Can you work these out from the model? Positions are in its coordinate system, mm. A direction names the side the tool comes from. Coordinates: 2 decimals unless noted, no trailing zeros. Order: outer loops, then holes, each group sorted by start corner. A loop starts at its lowest first (then second) coordinate and runs counter-clockwise, first axis right, second up. Notation, with made-up numbers: (78.5, 87.25) -> (121.5, 87.25) arc R20 ccw to (121.5, 98.25) -> close; hole circle Ø10 at (16.25, 42). An arc over 180 degrees is marked (long way). Answer as a JSON object with one key per item and string values. Group by question number.
(1) I want a section at C-C, the plane y = 22.5. List the corners of the cut face in (x, z) for me.
(2) I want a section at D-D, the plane y = 3. List the corners of the cut face in (x, z) for me (3 decimals), plus the area to 3 significant figures.
(3) For pin 1 (1.1 mm diameter, centred on x = 5, z = 4.5, fed in from -Y); pin 2 (0.5 mm diameter, centred on x = 5, z = 4.5, fed in from +Y); pin 3 (3 mm diameter, centred on x = 6, y = 3, fed in from +Z); pin 4 (3 mm diameter, centred on x = 4.5, y = 9.5, fed in from +Z), each with a flat end and sliding along its axis, tell me the tip position at first contact or that it passes through.
(4) I need wall thicknesses on line 1 (Y direction, x = 5, z = 1.65); line 2 (Y direction, x = 5, z = 3.35); line 3 (Y direction, x = 3, z = 1). Which ranges of each line are inside material? Lowest first, please.
(5) If we mould it in two halves opening along X, with no side actions, what happens to faces 6 (the cylindrical face through (9.699, 0.285, 2.028)), 7 (the cylindrical face through (4.792, 30.086, 1.521)), 8 (the flat face through (5, 6, 0))? For each: pulls with the +X half, pulls with the -X half, needs draft (parallel to the pull), parting line crosses it, or undercut.
(6) Which directions (+Z, -Z, +X, -X, +Y, -Y) give clear straight access to the entire face, cutting with the end or side of a thin tool? Please do faces 1 (the flat face through (5, 7, 4)), 2 (the cylindrical face through (5.86, 4.85, 1.52)), 3 (the cylindrical face through (7.586, 2.428, 3.507)), 4 (the cylindrical face through (5.07, 18.535, 0.301)), 5 (the cylindrical face through (9.699, 31.715, 2.028)).
(7) I want a section at B-B, the plane y = 28.5. List the corners of the cut face in (x, z) for me.
(8) I want a section at A-A, the plane x = 5. State how many separate pieces and enclosed holes the cut face has, plus the area to 3 significant figures.
from build123d import *

# Parameters (mm, degrees)
CROQUIS1_W              = 10
CROQUIS1_H              = 32
SALIENTE_EXTRUIR1_DEPTH = 8
CROQUIS2_R              = 1.6
CORTAR_EXTRUIR1_DEPTH   = 8
CROQUIS3_R              = 2.25
CORTAR_EXTRUIR2_DEPTH   = 10
REDONDEO1_R             = 1
CORTAR_EXTRUIR3_START   = -10
CROQUIS4_W              = 4
CROQUIS4_H              = 10
CORTAR_EXTRUIR3_DEPTH   = 10
REDONDEO2_R             = 3
REDONDEO3_R             = 1
CROQUIS5_R              = 2.8
CORTAR_EXTRUIR4_DEPTH   = 1


with BuildPart() as part:
    # Croquis1 → Saliente-Extruir1 (new body)
    with BuildSketch(Plane.XY):
        with Locations((5, 16)):
            Rectangle(CROQUIS1_W, CROQUIS1_H)
    extrude(amount=SALIENTE_EXTRUIR1_DEPTH)

    # Croquis2 → Cortar-Extruir1 (cut)
    with BuildSketch(Plane.XY.offset(8)):
        with Locations((5, 28.5)):
            Circle(CROQUIS2_R)
        with Locations((5, 3.5)):
            Circle(CROQUIS2_R)
    extrude(amount=-CORTAR_EXTRUIR1_DEPTH, mode=Mode.SUBTRACT)

    # Croquis3 → Cortar-Extruir2 (cut)
    with BuildSketch(Plane.ZY):
        with Locations((2.25, 16)):
            Circle(CROQUIS3_R)
        with BuildLine():
            ThreePointArc((0, 16.000000003), (0.659009743, 17.590990259), (2.25, 18.25))
            Line((2.25, 18.25), (0, 18.25))
            Line((0, 18.25), (0, 16.000000003))
        make_face()
        with BuildLine():
            ThreePointArc((2.25, 13.75), (0.659009741, 14.409009743), (0, 16.000000003))
            Line((0, 16.000000003), (0, 13.75))
            Line((0, 13.75), (2.25, 13.75))
        make_face()
    extrude(amount=-CORTAR_EXTRUIR2_DEPTH, mode=Mode.SUBTRACT)

    # Redondeo1
    redondeo1_edges = [part.edges().sort_by_distance(p)[0] for p in [
        (5, 13.75, 0),
        (5, 18.25, 0),
    ]]
    fillet(redondeo1_edges, radius=REDONDEO1_R)

    # Croquis4 → Cortar-Extruir3 (cut)
    with BuildSketch(Plane.ZY.offset(CORTAR_EXTRUIR3_START)):
        with Locations((6, 27)):
            Rectangle(CROQUIS4_W, CROQUIS4_H)
        with Locations((6, 5)):
            Rectangle(CROQUIS4_W, CROQUIS4_H)
    extrude(amount=CORTAR_EXTRUIR3_DEPTH, mode=Mode.SUBTRACT)

    # Redondeo2
    redondeo2_edges = [part.edges().sort_by_distance(p)[0] for p in [
        (5, 22, 8),
        (5, 10, 8),
    ]]
    fillet(redondeo2_edges, radius=REDONDEO2_R)

    # Redondeo3
    redondeo3_edges = [part.edges().sort_by_distance(p)[0] for p in [
        (0, 32, 2),
        (10, 32, 2),
        (10, 0, 2),
        (0, 0, 2),
    ]]
    fillet(redondeo3_edges, radius=REDONDEO3_R)

    # Croquis5 → Cortar-Extruir4 (cut)
    with BuildSketch(Plane.XY.offset(4)):
        with Locations((5, 28.5)):
            Circle(CROQUIS5_R)
        with Locations((5, 3.5)):
            Circle(CROQUIS5_R)
    extrude(amount=-CORTAR_EXTRUIR4_DEPTH, mode=Mode.SUBTRACT)


solid = part.part
Computed values:
{
 "1": {"outline": "(0, 0) -> (10, 0) -> (10, 4) -> (0, 4) -> close"},
 "2": {"outline": "(0, 0) -> (3.48, 0) -> (3.48, 3) -> (2.245, 3) -> (2.245, 4) -> (0, 4) -> close; (6.52, 0) -> (10, 0) -> (10, 4) -> (7.755, 4) -> (7.755, 3) -> (6.52, 3) -> close", "area": "25.4 mm2"},
 "3": {"pin 1": "stops at y = 0", "pin 2": "stops at y = 22", "pin 3": "stops at z = 3", "pin 4": "stops at z = 7.24"},
 "4": {"line 1": "y = 0 to 1.9, 5.1 to 13.75, 18.25 to 26.9, 30.1 to 32", "line 2": "y = 0 to 0.7, 6.3 to 14.04, 17.96 to 25.7, 31.3 to 32", "line 3": "y = 0 to 13.75, 18.25 to 32"},
 "5": {"face 6": "pulls with the +X half", "face 7": "undercut", "face 8": "needs draft"},
 "6": {"face 1": "+Z, +X, -X, -Y", "face 2": "+Z, -Z", "face 3": "+Z", "face 4": "-Z, +X, -X", "face 5": "+Z, -Z, +X, +Y"},
 "7": {"outline": "(0, 0) -> (3.4, 0) -> (3.4, 3) -> (2.2, 3) -> (2.2, 4) -> (0, 4) -> close; (6.6, 0) -> (10, 0) -> (10, 4) -> (7.8, 4) -> (7.8, 3) -> (6.6, 3) -> close"},
 "8": {"separate pieces": "3", "enclosed holes": "0", "area": "123 mm2"}
}
